```python
from build123d import *

# Parameters (mm, degrees)
SALIENTE_EXTRUIR1_DEPTH = 8.8
SALIENTE_EXTRUIR2_DEPTH = 10
CORTAR_EXTRUIR1_REACH   = 27
CROQUIS3_R              = 1.6
CORTAR_EXTRUIR2_DEPTH   = 11.8


with BuildPart() as part:
    # Croquis1 → Saliente-Extruir1 (new body)
    with BuildSketch(Plane.XY):
        Polygon((0, 0), (0, 15), (-25, 15), (-25, 6.2), (-18.8, 6.2), (-18.8, 0), align=None)
    extrude(amount=SALIENTE_EXTRUIR1_DEPTH)

    # Croquis2 → Saliente-Extruir2 (add)
    with BuildSketch(Plane.XY.offset(8.8)):
        Polygon((-8, 15), (-8, 6.2), (0, 6.2), (0, 0), (-8, 0), (-18.8, 0), (-18.8, 6.2), (-25, 6.2), (-25, 15), align=None)
    extrude(amount=SALIENTE_EXTRUIR2_DEPTH)

    # Croquis3 → Cortar-Extruir1 (cut, up to next)
    with BuildSketch(Plane(origin=(0, 0, 0), x_dir=(0, 0, -1), z_dir=(1, 0, 0)), mode=Mode.PRIVATE) as cortar_extruir1_sk1:
        with Locations((-4.1, 3.1)):
            Circle(CROQUIS3_R)
    cortar_extruir1_tool1 = extrude(cortar_extruir1_sk1.sketch, amount=-CORTAR_EXTRUIR1_REACH, mode=Mode.PRIVATE) & part.part
    add(cortar_extruir1_tool1.solids().sort_by_distance((0, 3.1, 4.1))[0], mode=Mode.SUBTRACT)

    # Croquis4 → Cortar-Extruir2 (cut)
    with BuildSketch(Plane(origin=(0, 0, 0), x_dir=(0, 0, -1), z_dir=(1, 0, 0))):
        Polygon((-0.809103466, 3.1), (-2.454551733, 5.95), (-5.745448267, 5.95), (-7.390896534, 3.1), (-5.745448267, 0.25), (-2.454551733, 0.25), align=None)
    extrude(amount=-CORTAR_EXTRUIR2_DEPTH, mode=Mode.SUBTRACT)


solid = part.part
```
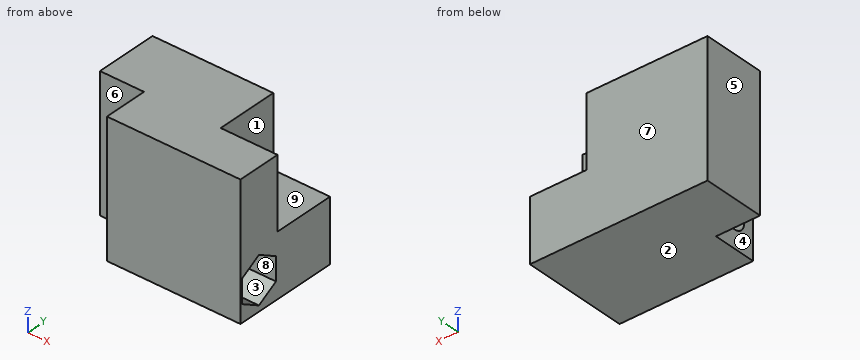
Part model, mm, in its own coordinate system. Face numbers are marked on the shaded views. A direction names the side the tool comes from. Round coordinates to 2 decimals unless told otherwise and drop trailing zeros. Write each loop counter-clockwise with the first axis right and the second up, starting at its lowest first coordinate (ties: lowest second). Pieces come first, ordered by that corner, then holes. Notation, with made-up numbers: M 40,-31.5 L 83,-31.5 A21 cw 83,-9.5 Z; hole C 83.25,83 d7. An arc over 180 degrees is marked long. Answer as CSV lines item,"result". Start each with the question number.
1) Band-saw the part on B-B (z = 4.1). List the corners of the cut face in (x, y), then the cut area to 3 significant figures.
2) Mould opens along Y. For the marked faces 6, 7, 8 and 9 say: +Y half, -Y half, draft (parallel to the pull), parting line (faces both ways), or undercut.
3) Drop flat-ended pins along their axis: pin 1 (2.5 mm diameter, centred on x = -5, z = 12, fed in from +Y); pin 2 (1 mm diameter, centred on y = 4.5, z = 12, fed in from -X); pin 3 (1.9 mm diameter, centred on x = -21, z = 6.5, fed in from -Y). Give the stop position or say it passes through.
4) Band-saw the part on D-D (z = 17). List the corners of the cut face in (x, y), then the cut area to 3 significant figures.
5) Band-saw the part on A-A (x = -17). List the corners of the cut face in (y, z).
6) Drill centre lines: L1, parallel to Y at x = -17, z = 4.1; L2, parallel to Y at x = -20, z = 7.5; L3, parallel to X at y = 2.5, z = 11.75. Where is each one in solid material? Low to high.
7) Band-saw the part on C-C (y = 2.25). List the corners of the cut face in (x, z), then the cut area to 3 significant figures.
8) Which spindle directions (+Z, -Z, +X, -X, +Y, -Y) get a long thin tool onto all of the face, cutting with end or side? Do the marked faces 1, 2, 3, 4 and 5. Say none if no direction does.
Worked out:
1,outline,"M -25,6.2 L -18.8,6.2 L -18.8,4.7 L -11.8,4.7 L -11.8,5.95 L 0,5.95 L 0,15 L -25,15 Z; M -18.8,0 L 0,0 L 0,0.25 L -11.8,0.25 L -11.8,1.5 L -18.8,1.5 Z"
1,area,"247 mm²"
2,face 6,"-Y half"
2,face 7,"+Y half"
2,face 8,"undercut"
2,face 9,"draft"
3,pin 1,"y = 6.2"
3,pin 2,"x = -18.8"
3,pin 3,"y = 6.2"
4,outline,"M -25,6.2 L -18.8,6.2 L -18.8,0 L 0,0 L 0,6.2 L -8,6.2 L -8,15 L -25,15 Z"
4,area,"266 mm²"
5,outline,"M 0,0 L 15,0 L 15,18.8 L 0,18.8 Z; hole C 3.1,4.1 d3.2"
6,L1,"0 to 1.5, 4.7 to 15"
6,L2,"6.2 to 15"
6,L3,"-18.8 to 0"
7,outline,"M -18.8,0 L 0,0 L 0,1.3 L -11.8,1.3 L -11.8,2.74 L -18.8,2.74 Z; M -18.8,5.46 L -11.8,5.46 L -11.8,6.9 L 0,6.9 L 0,18.8 L -18.8,18.8 Z"
7,area,"268 mm²"
8,face 1,"+Z, +X, +Y"
8,face 2,"-Z, +X, -X, +Y, -Y"
8,face 3,"+X"
8,face 4,"+Z, -Z, -X, -Y"
8,face 5,"+Z, -Z, -X, +Y, -Y"
